from build123d import *

# Parameters (mm, degrees)
SKETCH1_R           = 35
BOSS_EXTRUDE1_DEPTH = 75
SKETCH2_W           = 40
SKETCH2_H           = 40
CUT_EXTRUDE1_DEPTH  = 90.86100377805714
BOSS_EXTRUDE2_START = -10
BOSS_EXTRUDE2_DEPTH = 55
SKETCH5_R           = 35.00000000000001
BOSS_EXTRUDE3_DEPTH = 100
SKETCH8_R           = 25.000000000000007
BOSS_EXTRUDE5_DEPTH = 50
FILLET1_R           = 10
FILLET2_R           = 10


with BuildPart() as part:
    # Sketch1 → Boss-Extrude1 (new body)
    with BuildSketch(Plane(origin=(0, 0, 0), x_dir=(1, 0, 0), z_dir=(0, 1, 0))):
        with Locations(Location((0, 0, 0), (0, 0, 270))):
            Circle(SKETCH1_R)
    extrude(amount=BOSS_EXTRUDE1_DEPTH)

    # Sketch2 → Cut-Extrude1 (cut, through all)
    with BuildSketch(Plane(origin=(0, 75, 0), x_dir=(1, 0, 0), z_dir=(0, 1, 0))):
        Rectangle(SKETCH2_W, SKETCH2_H)
    extrude(amount=-CUT_EXTRUDE1_DEPTH, mode=Mode.SUBTRACT)

    # Sketch3 → Boss-Extrude2 (add)
    with BuildSketch(Plane(origin=(0, 75, 0), x_dir=(1, 0, 0), z_dir=(0, 1, 0)).offset(BOSS_EXTRUDE2_START)):
        Polygon((228.72281323269016, -19.99999999999999), (28.72281323269015, -20.000000000000014), (28.72281323269015, 19.999999999999982), (228.72281323269016, 20.00000000000001), align=None)
    extrude(amount=-BOSS_EXTRUDE2_DEPTH)

    # Sketch5 → Boss-Extrude3 (add)
    with BuildSketch(Plane(origin=(-2.78e-15, 0, -19.99999999999998), x_dir=(-1, 0, 1.4e-16), z_dir=(-1.4e-16, 0, -1))):
        with Locations((-250.37344832730113, 37.49999999999998)):
            Circle(SKETCH5_R)
    extrude(amount=-BOSS_EXTRUDE3_DEPTH)

    # Sketch8 → Boss-Extrude5 (add)
    with BuildSketch(Plane.XY.offset(80.00000000000003)):
        with Locations((250.37344832730113, 37.49999999999998)):
            Circle(SKETCH8_R)
    extrude(amount=BOSS_EXTRUDE5_DEPTH)

    # Fillet1
    fillet1_edges = [part.edges().sort_by_distance(p)[0] for p in [
        (128.72281323269016, 10, -19.999999999999996),
        (128.72281323269016, 10, 20.000000000000004),
        (128.72281323269016, 65, 20.000000000000004),
        (128.72281323269016, 65, -19.999999999999996),
    ]]
    fillet(fillet1_edges, radius=FILLET1_R)

    # Fillet2
    fillet2_edges = [part.edges().sort_by_distance(p)[0] for p in [
        (285.37344832730116, 37.49999999999991, -20.00000000000001),
    ]]
    fillet(fillet2_edges, radius=FILLET2_R)


with BuildPart() as part_1:
    # Body-Move/Copy1: moved
    add(part.part.moved(Location((-250, -37.5, 0))))


solid = part_1.part
Source: CAD feature listing. Evaluate the final solid. Frame: model axes, mm. A direction names the side the tool comes from. Coordinates: 2 decimals unless noted, no trailing zeros. Loops run counter-clockwise (first coordinate to the right, second up) from the corner with the lowest first, then second, coordinate; pieces in that order, holes last. Notation, with made-up numbers: (50, 45.5) - (87, 45.5) arc R22 ccw to (87, 71.5) - close; hole circle Ø10 at (-29, -38). An arc over 180 degrees is marked (long way). Return JSON: item names as keys, results as strings.
Q1. Section B-B, the plane z = 0. Return loops of the section in (x, y).
Results:
{"outline": "(-285, -37.5) - (-270, -37.5) - (-270, 37.5) - (-285, 37.5) - close; (-230, -37.5) - (-215, -37.5) - (-215, -27.5) - (-21.28, -27.5) arc R35 ccw (long way) to (-21.28, 27.5) - (-215, 27.5) - (-215, 37.5) - (-230, 37.5) - close"}
Q2. Material intervals for line 1 along Y through (x, z) = (-126, 4.5); line 2 along Z through (x, y) = (-126, 18.5); line 3 along Z through (x, y) = (2, -22), sorted ascending.
Results:
{"line 1": "-27.5 to 27.5", "line 2": "-19.95 to 19.95", "line 3": "-20 to 130"}
Q3. Contact query for flat-ended pins moving along their axis: P1, Ø20, axis at x = -254, y = -15, coming from the +Z side; P2, Ø22, axis at x = -84.5, z = -0.5, coming from the -Y side; P3, Ø1, axis at x = -42.5, z = 18.5, coming from the +Y side. Output: stop coordinate, or through.
Results:
{"P1": "z = 35", "P2": "y = -27.5", "P3": "y = 23.5"}
Q4. Section C-C, the plane x = -184.5. Return loops of the section in (y, z), plus the area to 3 significant figures.
Results:
{"outline": "(-27.5, -10) arc R10 ccw to (-17.5, -20) - (17.5, -20) arc R10 ccw to (27.5, -10) - (27.5, 10) arc R10 ccw to (17.5, 20) - (-17.5, 20) arc R10 ccw to (-27.5, 10) - close", "area": "2,110 mm2"}
Q5. Section A-A, the plane x = -250. Return loops of the section in (y, z).
Results:
{"outline": "(-37.5, -35) - (37.5, -35) - (37.5, -20) - (-37.5, -20) - close; (-37.5, 20) - (37.5, 20) - (37.5, 35) - (-37.5, 35) - close"}
Q6. Section D-D, the plane z = 55. Return loops of the section in (x, y), plus the area to 3 significant figures.
Results:
{"outline": "circle Ø70 at (0.37, 0)", "area": "3,850 mm2"}
Q7. Access query for faces 1 (the cylindrical face through (35.34, 1.54, 34.37)), 2 (the flat face through (-270, 1, 0)), 3 (the flat face through (-118, -27.5, 0)), 4 (the cylindrical face through (-122.68, 24.65, 16.99)). Directions: +Z, -Z, +X, -X, +Y, -Y. A direction counts if a zero-diameter tool reaches every point of the face in a straight line with its end or side. Return the directions, or none.
Results:
{"face 1": "+Z", "face 2": "+Y, -Y", "face 3": "+Z, -Z, -Y", "face 4": "+Z, +Y"}
Q8. Mould query, pull axis X, two halves, no side actions, for faces 5 (the cylindrical face through (11.91, -22.18, 104.65)), 6 (the flat face through (-124, 0, 20)), 7 (the flat face through (-250, -37.5, 23)). Classes: released by +X, released by -X, zero draft, split by the parting line, or undercut.
Results:
{"face 5": "split by the parting line", "face 6": "undercut", "face 7": "zero draft"}
